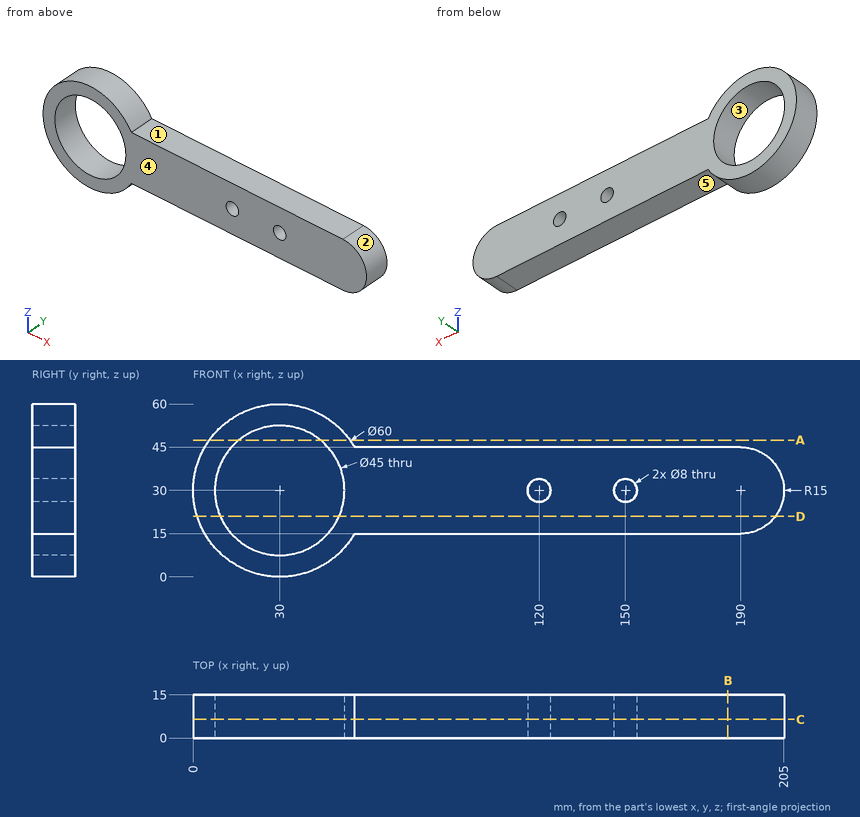
Check sheet for the drawn part. Datum: minimum x, y, z corner. Units: mm. A direction names the side the tool comes from. Round coordinates to 2 decimals unless told otherwise and drop trailing zeros. Order: outer loops, then holes, each group sorted by start corner. A loop starts at its lowest first (then second) coordinate and runs counter-clockwise, first axis right, second up. Notation, with made-up numbers: (-5.5, 2.5) - (52.5, 2.5) arc R14 ccw to (52.5, 23.5) - close; hole circle Ø5 at (61, 12). An arc over 180 degrees is marked (long way). Use a Markdown table: item, result. Add a question column.
(1) Sectioned sample at C-C, the plane y = 6.5. Enter the section's corners in (x, z).
(2) Depth check by flat-ended pin: pin 1 (8 mm diameter, centred on x = 86.5, y = 8.5, fed in from -Z); pin 2 (4 mm diameter, centred on y = 9, z = 28.5, fed in from +X); pin 3 (2 mm diameter, centred on y = 5, z = 25.5, fed in from +X); pin 4 (1.5 mm diameter, centred on y = 6, z = 15.5, fed in from -X). Enter the tip coordinate at first touch or a pass-through.
(3) Release check for a two-part mould opening along Z. For the marked faces 1, 2 and 3 record: pulls with the +Z half, pulls with the -Z half, needs draft (parallel to the pull), parting line crosses it, or undercut.
(4) Sectioned sample at B-B, the plane x = 185.5. Enter the section's corners in (y, z), and give its area (3 significant figures).
(5) Tool access check on the marked faces 4 and 5. Record the directions out of +Z, -Z, +X, -X, +Y, -Y that give a thin tool (end or side, any length) a straight path to the whole face; none if there is none.
(6) Sectioned sample at A-A, the plane z = 47.5. Enter the section's corners in (x, y).
(7) Sectioned sample at D-D, the plane z = 21. Enter the section's corners in (x, y), and give its area (3 significant figures).
(8) Material ranges on line 1 along Z through (x, y) = (88.5, 2.75); line 2 along X through (y, z) = (6, 27.5); line 3 along X through (y, z) = (12, 27), recorded low to high. Write a range as [from, to].
Answers below:
| question | item | result |
|---|---|---|
| 1 | outline | (55.98, 15) - (190, 15) arc R15 ccw to (190, 45) - (55.98, 45) arc R30 ccw (long way) to start; hole circle Ø45 at (30, 30); hole circle Ø8 at (120, 30); hole circle Ø8 at (150, 30) |
| 2 | pin 1 | z = 15 |
| 2 | pin 2 | x = 205 |
| 2 | pin 3 | x = 204.59 |
| 2 | pin 4 | x = 3.34 |
| 3 | face 1 | pulls with the +Z half |
| 3 | face 2 | parting line crosses it |
| 3 | face 3 | undercut |
| 4 | outline | (0, 15) - (15, 15) - (15, 45) - (0, 45) - close |
| 4 | area | 450 mm² |
| 5 | face 4 | +Z, -Z, +X, -X, -Y |
| 5 | face 5 | -Z, +X, +Y, -Y |
| 6 | outline | (5.63, 0) - (15.86, 0) - (15.86, 15) - (5.63, 15) - close; (44.14, 0) - (54.37, 0) - (54.37, 15) - (44.14, 15) - close |
| 7 | outline | (1.38, 0) - (9.38, 0) - (9.38, 15) - (1.38, 15) - close; (50.62, 0) - (202, 0) - (202, 15) - (50.62, 15) - close |
| 7 | area | 2,390 mm² |
| 8 | line 1 | [15, 45] |
| 8 | line 2 | [0.1, 7.64], [52.36, 116.88], [123.12, 146.88], [153.12, 204.79] |
| 8 | line 3 | [0.15, 7.7], [52.3, 117.35], [122.65, 147.35], [152.65, 204.7] |
